Input: dimensioned drawing with shaded views. Units: mm. Origin: part minimum x, y, z. A direction names the side the tool comes from. Coordinates: 2 decimals unless noted, no trailing zeros. Write each loop counter-clockwise with the first axis right and the second up, starting at its lowest first coordinate (ties: lowest second). Pieces come first, ordered by that corner, then holes. Notation, with made-up numbers: M 51,7.5 L 72,7.5 A33 ccw 72,39.5 Z; hole C -3,-16.75 d2. An arc over 180 degrees is marked long. Use one line per item in the form item = value.
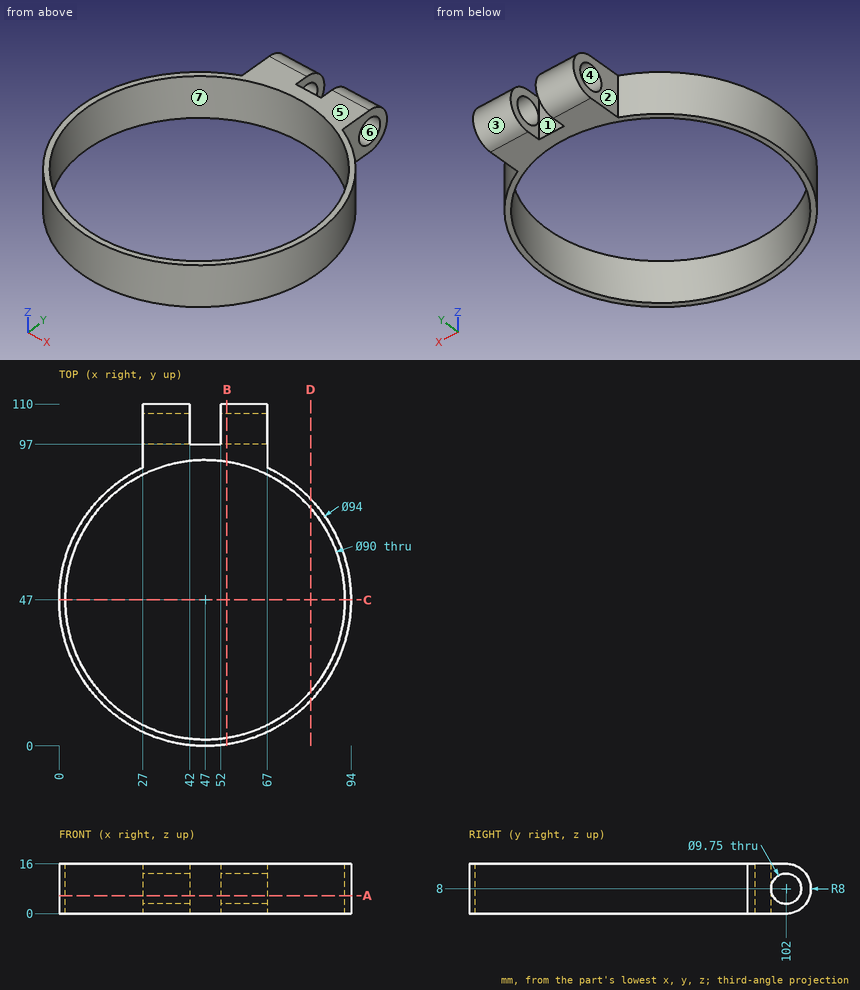
(1) Line query: probe 1 along X at (y, z) = (47, 7.5); probe 2 along Z at (x, y) = (62.5, 102) (3 decimals); probe 3 along Y at (x, z) = (46.5, 11.5). Output: solid intervals per line, ascending.
Computed:
probe_1 = 0 to 2, 92 to 94
probe_2 = 0 to 3.125, 12.875 to 16
probe_3 = 0 to 2, 92 to 97
(2) Section query B-B on x = 54. Return the cut outline in (y, z) (3 decimals), plus the area to 3 significant figures.
Computed:
outline = M 0.524,0 L 2.548,0 L 2.548,16 L 0.524,16 Z; M 91.452,0 L 102,0 A8 ccw 102,16 L 91.452,16 Z; hole C 102,8 d9.75
area = 227 mm^2
(3) Section query A-A on z = 5.75. Return the cut outline in (x, y).
Computed:
outline = M 27,89.53 A47 ccw long 67,89.53 L 67,97.68 L 52,97.68 L 52,97 L 42,97 L 42,97.68 L 27,97.68 Z; M 27,106.32 L 42,106.32 L 42,109.68 L 27,109.68 Z; M 52,106.32 L 67,106.32 L 67,109.68 L 52,109.68 Z; hole C 47,47 d90
(4) Pull-direction query (Z, two-part tool) for the marked faces 4, 5, 6 and 7; classes: pulls with the +Z half, pulls with the -Z half, needs draft (parallel to the pull), parting line crosses it, or undercut.
Computed:
face_4 = undercut
face_5 = pulls with the +Z half
face_6 = undercut
face_7 = needs draft
(5) Section query D-D on x = 81. Return the cut outline in (y, z).
Computed:
outline = M 14.55,0 L 17.52,0 L 17.52,16 L 14.55,16 Z; M 76.48,0 L 79.45,0 L 79.45,16 L 76.48,16 Z
(6) Section query C-C on y = 47. Return the cut outline in (x, z), plus the area to 3 significant figures.
Computed:
outline = M 0,0 L 2,0 L 2,16 L 0,16 Z; M 92,0 L 94,0 L 94,16 L 92,16 Z
area = 64.0 mm^2
(7) First-contact query: pin 1 Ø5 at (x, z) = (37.5, 5.5) entering from -Y; pin 2 Ø8 at (y, z) = (102, 8) entering from -X; pin 3 Ø5 at (x, z) = (29, 11) entering from +Y; pin 4 Ø5 at (y, z) = (99, 10) entering from -X. Flat tips, straight axial feed; report the tip coordinate or a pass-through.
Computed:
pin_1 = 0.52
pin_2 = through
pin_3 = 109.98
pin_4 = 27
(8) Set-up query: the marked faces 1, 2 and 3. Return all of +Z, -Z, +X, -X, +Y, -Y with unobstructed straight access to the full face (end or side cutting, diameter ignored); none if empty.
Computed:
face_1 = +Z, -Z, +Y
face_2 = +Z, -Z, -X, +Y
face_3 = +X, -X, +Y
